```python
from build123d import *

# Parameters (mm, degrees)
SKETCH1_W           = 11
SKETCH1_H           = 11
BOSS_EXTRUDE1_DEPTH = 3.7
FILLET1_R           = 1
SKETCH2_W           = 3.85
SKETCH2_H           = 3.85
CUT_EXTRUDE1_DEPTH  = 2
SKETCH4_R           = 2.2
BOSS_EXTRUDE2_DEPTH = 4
BOSS_EXTRUDE3_DEPTH = 2
SKETCH3_R           = 1.2
CUT_EXTRUDE2_DEPTH  = 17.726924403
CUT_EXTRUDE3_DEPTH  = 16.90565937
SKETCH8_R           = 2.2
SKETCH8_R_2         = 1.2
BOSS_EXTRUDE4_DEPTH = 4


with BuildPart() as part:
    # Sketch1 → Boss-Extrude1 (new body)
    with BuildSketch(Plane(origin=(0, 0, 0), x_dir=(1, 0, 0), z_dir=(0, 1, 0))):
        Rectangle(SKETCH1_W, SKETCH1_H)
    extrude(amount=BOSS_EXTRUDE1_DEPTH)

    # Fillet1
    fillet1_edges = [part.edges().sort_by_distance(p)[0] for p in [
        (5.5, 1.85, 5.5),
        (-5.5, 1.85, 5.5),
        (-5.5, 1.85, -5.5),
        (5.5, 1.85, -5.5),
    ]]
    fillet(fillet1_edges, radius=FILLET1_R)

    # Sketch2 → Cut-Extrude1 (cut)
    with BuildSketch(Plane(origin=(0, 3.7, 0), x_dir=(1, 0, 0), z_dir=(0, 1, 0))):
        with Locations((-2.825, 0)):
            Rectangle(SKETCH2_W, SKETCH2_H)
        with Locations((2.825, 0)):
            Rectangle(SKETCH2_W, SKETCH2_H)
    extrude(amount=-CUT_EXTRUDE1_DEPTH, mode=Mode.SUBTRACT)

    # Sketch4 → Boss-Extrude2 (add)
    with BuildSketch(Plane(origin=(0, 0, 0), x_dir=(-1, 0, 0), z_dir=(0, -1, 0))):
        with Locations(Location((2.825, 0, 0), (0, 0, 90))):
            Circle(SKETCH4_R)
        with Locations(Location((-2.825, 0, 0), (0, 0, 90))):
            Circle(SKETCH4_R)
    extrude(amount=BOSS_EXTRUDE2_DEPTH)

    # Sketch5 → Boss-Extrude3 (add)
    with BuildSketch(Plane(origin=(0, -4, 0), x_dir=(-1, 0, 0), z_dir=(0, -1, 0))):
        with BuildLine():
            Line((9.5, 10.5), (-9.5, 10.5))
            ThreePointArc((-9.5, 10.5), (-10.207106781, 10.207106781), (-10.5, 9.5))
            Line((-10.5, 9.5), (-10.5, -9.5))
            ThreePointArc((-10.5, -9.5), (-10.207106781, -10.207106781), (-9.5, -10.5))
            Line((-9.5, -10.5), (9.5, -10.5))
            ThreePointArc((9.5, -10.5), (10.207106781, -10.207106781), (10.5, -9.5))
            Line((10.5, -9.5), (10.5, 9.5))
            ThreePointArc((10.5, 9.5), (10.207106781, 10.207106781), (9.5, 10.5))
        make_face()
    extrude(amount=-BOSS_EXTRUDE3_DEPTH)

    # Sketch3 → Cut-Extrude2 (cut, through all)
    with BuildSketch(Plane(origin=(0, 3.7, 0), x_dir=(1, 0, 0), z_dir=(0, 1, 0))):
        with Locations(Location((-2.825, 0, 0), (0, 0, 270))):
            Circle(SKETCH3_R)
        with Locations(Location((2.825, 0, 0), (0, 0, 270))):
            Circle(SKETCH3_R)
    extrude(amount=-CUT_EXTRUDE2_DEPTH, mode=Mode.SUBTRACT)

    # Sketch7 → Cut-Extrude3 (cut, through all)
    with BuildSketch(Plane(origin=(0, -2, 0), x_dir=(1, 0, 0), z_dir=(0, 1, 0))):
        with BuildLine():
            Line((0, -9.085786438), (1.414213562, -10.5))
            Line((1.414213562, -10.5), (3.889087297, -8.025126266))
            ThreePointArc((3.889087297, -8.025126266), (4.035533906, -7.671572875), (3.889087297, -7.318019485))
            Line((3.889087297, -7.318019485), (3.181980515, -6.610912703))
            ThreePointArc((3.181980515, -6.610912703), (2.828427125, -6.464466094), (2.474873734, -6.610912703))
            Line((2.474873734, -6.610912703), (0, -9.085786438))
        make_face()
        with BuildLine():
            Line((-3.889087297, -8.025126266), (-1.414213562, -10.5))
            Line((-1.414213562, -10.5), (0, -9.085786438))
            Line((0, -9.085786438), (-2.474873734, -6.610912703))
            ThreePointArc((-2.474873734, -6.610912703), (-2.828427125, -6.464466094), (-3.181980515, -6.610912703))
            Line((-3.181980515, -6.610912703), (-3.889087297, -7.318019485))
            ThreePointArc((-3.889087297, -7.318019485), (-4.035533906, -7.671572875), (-3.889087297, -8.025126266))
        make_face()
        Polygon((-1.414213562, -10.5), (1.414213562, -10.5), (0, -9.085786438), align=None)
    extrude(amount=-CUT_EXTRUDE3_DEPTH, mode=Mode.SUBTRACT)

    # Sketch8 → Boss-Extrude4 (add)
    # profile 1 of 2: a face of its own
    with BuildSketch(Plane.XZ.offset(4)):
        with Locations(Location((-2.825, 0, 0), (0, 0, 90))):
            Circle(SKETCH8_R)
        with Locations(Location((-2.825, 0, 0), (0, 0, 90))):
            Circle(SKETCH8_R_2, mode=Mode.SUBTRACT)
    # profile 2 of 2: a face of its own
    with BuildSketch(Plane.XZ.offset(4)):
        with Locations(Location((2.825, 0, 0), (0, 0, 90))):
            Circle(SKETCH8_R)
        with Locations(Location((2.825, 0, 0), (0, 0, 90))):
            Circle(SKETCH8_R_2, mode=Mode.SUBTRACT)
    extrude(amount=BOSS_EXTRUDE4_DEPTH)


solid = part.part
```
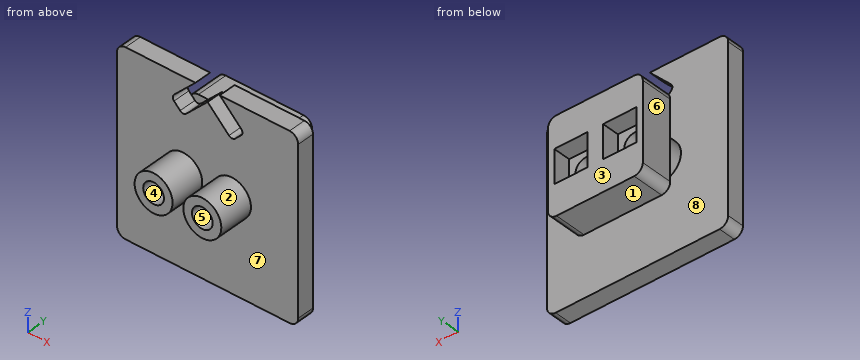
Could you check a few things on this model? Use its own coordinates, in mm. Face numbers are marked on the shaded views. A direction names the side the tool comes from. Round coordinates to 2 decimals unless told otherwise and drop trailing zeros. Loops run counter-clockwise (first coordinate to the right, second up) from the corner with the lowest first, then second, coordinate; pieces in that order, holes last. Notation, with made-up numbers: (63, 22) - (80, 22) arc R28 ccw to (80, 58) - close; hole circle Ø9 at (57, 8.25). An arc over 180 degrees is marked (long way). Use CSV: the item, a comma, the result in double quotes.
Item 1: If we section it at B-B on y = -3: List the corners of the cut face in (x, z) for me (3 decimals).
Here are the results:
outline,"(-10.5, -9.5) arc R1 ccw to (-9.5, -10.5) - (9.5, -10.5) arc R1 ccw to (10.5, -9.5) - (10.5, 9.5) arc R1 ccw to (9.5, 10.5) - (1.414, 10.5) - (3.889, 8.025) arc R0.5 cw to (3.889, 7.318) - (3.182, 6.611) arc R0.5 cw to (2.475, 6.611) - (0, 9.086) - (-2.475, 6.611) arc R0.5 cw to (-3.182, 6.611) - (-3.889, 7.318) arc R0.5 cw to (-3.889, 8.025) - (-1.414, 10.5) - (-9.5, 10.5) arc R1 ccw to (-10.5, 9.5) - close; hole circle Ø2.4 at (-2.825, 0); hole circle Ø2.4 at (2.825, 0)"
Item 2: Will these pins go through, and if not, where does the flat tip stop? pin 1 (1.5 mm diameter, centred on x = 3, z = 6, fed in from -Y); pin 2 (4 mm diameter, centred on y = 1.5, z = -2, fed in from -X); pin 3 (3 mm diameter, centred on x = 1.5, y = 2, fed in from +Z).
Here are the results:
pin 1,"stops at y = -4"
pin 2,"stops at x = -5.5"
pin 3,"stops at z = 5.5"
Item 3: If we section it at A-A on z = 2.75: List the corners of the cut face in (x, y) for me.
Here are the results:
outline,"(-10.5, -4) - (10.5, -4) - (10.5, -2) - (-10.5, -2) - close; (-5.5, 0) - (5.5, 0) - (5.5, 3.7) - (-5.5, 3.7) - close"
Item 4: For the marked faces 5, 6, 7 and 8, which set-ups out of +Z, -Z, +X, -X, +Y, -Y let a thin tool reach every point of the face, with its end or its side?
Here are the results:
face 5,"+Y, -Y"
face 6,"+Z, -Z, -X, +Y"
face 7,"-Y"
face 8,"none"
Item 5: If we section it at D-D on y = -5: List the corners of the cut face in (x, z) for me (3 decimals), then the cut area to 3 significant figures.
Here are the results:
outline,"circle Ø4.4 at (-2.825, 0); circle Ø4.4 at (2.825, 0); hole circle Ø2.4 at (-2.825, 0); hole circle Ø2.4 at (2.825, 0)"
area,"21.4 mm²"
Item 6: If we mould it in two halves opening along Z, with no side actions, what happens to the marked faces 1, 2, 3 and 4? For each: pulls with the +Z half, pulls with the -Z half, needs draft (parallel to the pull), parting line crosses it, or undercut.
Here are the results:
face 1,"pulls with the -Z half"
face 2,"parting line crosses it"
face 3,"needs draft"
face 4,"undercut"
Item 7: I need wall thicknesses on L1, parallel to Y at x = -2, z = 2.5; L2, parallel to X at y = -3, z = 0 (3 decimals); L3, parallel to X at y = -1, z = 0 (3 decimals). Which ranges of each line are inside material? Lowest first, please. Write a range as [from, to].
Here are the results:
L1,"y = [-4, -2], [0, 3.7]"
L2,"x = [-10.5, -4.025], [-1.625, 1.625], [4.025, 10.5]"
L3,"x = [-5.025, -4.025], [-1.625, -0.625], [0.625, 1.625], [4.025, 5.025]"
